For this review, use the dimensioned drawing (mm, ordinates from the lowest corner) and the shaded views. A direction names the side the tool comes from. Coordinates: 2 decimals unless noted, no trailing zeros. Order: outer loops, then holes, each group sorted by start corner. A loop starts at its lowest first (then second) coordinate and runs counter-clockwise, first axis right, second up. Notation, with made-up numbers: M 65.25,-30.75 L 113.25,-30.75 A18 cw 113.25,-23.75 Z; hole C 37.5,69 d11. An arc over 180 degrees is marked long. Answer in a Markdown table with one row per item.
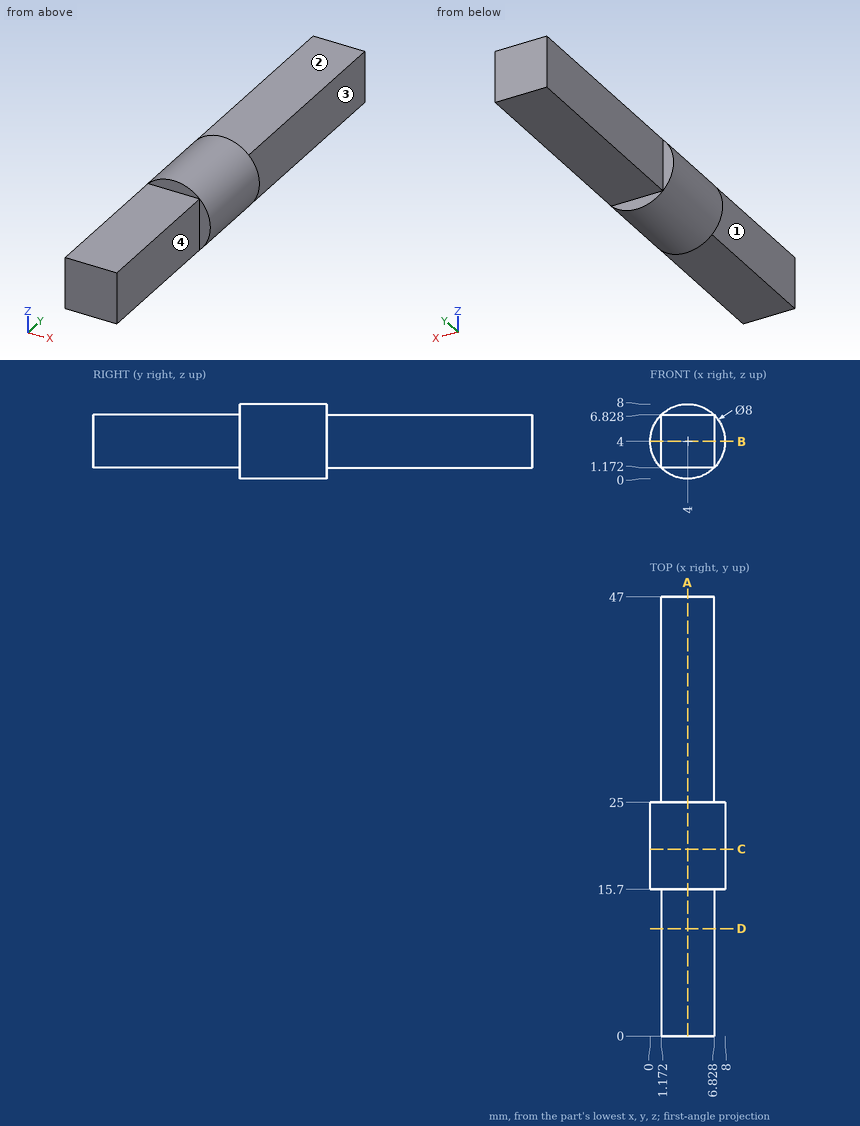
(1) Add section B-B, the plane z = 4. Give the boundary of the cut face in (x, y), and give its area (3 significant figures).
Return value:
| item | result |
|---|---|
| outline | M 0,15.7 L 1.17,15.7 L 1.17,0 L 6.83,0 L 6.83,15.7 L 8,15.7 L 8,25 L 6.83,25 L 6.83,47 L 1.17,47 L 1.17,25 L 0,25 Z |
| area | 288 mm2 |
(2) Insertion check: pin 1 Ø1.7 at (x, y) = (5, 31.5) entering from -Z; pin 2 Ø0.9 at (x, z) = (0.5, 4) entering from +Y; pin 3 Ø4.5 at (y, z) = (9.5, 5.5) entering from -X. Each pin has a flat end and moves straight along its axis. Give the tip position at first contact, or say it passes through.
Return value:
| item | result |
|---|---|
| pin 1 | stops at z = 1.17 |
| pin 2 | stops at y = 25 |
| pin 3 | stops at x = 1.17 |
(3) For the marked faces 1, 2, 3 and 4, list the 3-axis set-ups (+Z, -Z, +X, -X, +Y, -Y) from which the entire face can be reached by the end or side of a thin tool; tool diameter is ignored.
Return value:
| item | result |
|---|---|
| face 1 | +Z, -Z, -X, -Y |
| face 2 | +Z, +X, -X, +Y |
| face 3 | +Z, -Z, +X, +Y |
| face 4 | +Z, -Z, +X, -Y |
(4) Add section A-A, the plane x = 4. Give the boundary of the cut face in (y, z).
Return value:
| item | result |
|---|---|
| outline | M 0,1.17 L 15.7,1.17 L 15.7,0 L 25,0 L 25,1.17 L 47,1.17 L 47,6.83 L 25,6.83 L 25,8 L 15.7,8 L 15.7,6.83 L 0,6.83 Z |
(5) For line 1 along X through (y, z) = (39, 5); line 2 along Y through (x, z) = (4, 7.5), list the stretches that pass through material, from the lowest coordinate up. Write a range as from..to.
Return value:
| item | result |
|---|---|
| line 1 | x = 1.17..6.83 |
| line 2 | y = 15.7..25 |
(6) Add section D-D, the plane y = 11.5. Give the boundary of the cut face in (x, z), and give its area (3 significant figures).
Return value:
| item | result |
|---|---|
| outline | M 1.17,1.17 L 6.83,1.17 L 6.83,6.83 L 1.17,6.83 Z |
| area | 32.0 mm2 |
(7) Add section C-C, the plane y = 20. Give the boundary of the cut face in (x, z).
Return value:
| item | result |
|---|---|
| outline | C 4,4 d8 |
